from build123d import *

# Parameters (mm, degrees)
PAD001_DEPTH = 2.1
THICKNESS_T  = -0.5
FILLET_R     = 0.3
FILLET001_R  = 0.1


with BuildPart() as part:
    # Sketch001 → Pad001 (new body)
    with BuildSketch(Plane.XY):
        Polygon((5, 18.8), (34, 18.8), (34, 1.2), (1.2, 1.2), (1.2, 15.3), (5, 15.3), align=None)
    extrude(amount=PAD001_DEPTH)

    # Thickness
    thickness_openings = [part.faces().sort_by_distance(p)[0] for p in [
        (17.941945, 9.833744, 0),
    ]]
    offset(amount=THICKNESS_T, openings=thickness_openings, kind=Kind.INTERSECTION)

    # Fillet
    fillet_edges = [part.edges().sort_by_distance(p)[0] for p in [
        (1.2, 1.2, 1.05),
        (34, 1.2, 1.05),
        (34, 18.8, 1.05),
        (5, 18.8, 1.05),
        (5, 15.3, 1.05),
        (1.2, 15.3, 1.05),
        (1.2, 8.25, 2.1),
        (17.6, 1.2, 2.1),
        (34, 10, 2.1),
        (19.5, 18.8, 2.1),
        (5, 17.05, 2.1),
        (3.1, 15.3, 2.1),
    ]]
    fillet(fillet_edges, radius=FILLET_R)

    # Fillet001
    fillet001_edges = [part.edges().sort_by_distance(p)[0] for p in [
        (1.7, 1.7, 0.8),
        (33.5, 1.7, 0.8),
        (33.5, 18.3, 0.8),
        (5.5, 18.3, 0.8),
        (5.5, 14.8, 0.8),
        (1.7, 14.8, 0.8),
        (1.7, 8.25, 1.6),
        (3.6, 14.8, 1.6),
        (5.5, 16.55, 1.6),
        (19.5, 18.3, 1.6),
        (17.6, 1.7, 1.6),
        (33.5, 10, 1.6),
    ]]
    fillet(fillet001_edges, radius=FILLET001_R)


solid = part.part
The listing builds one solid part. Answer for the finished solid, in the listing's coordinates (mm). A direction names the side the tool comes from. Coordinates: 2 decimals unless noted, no trailing zeros. Loops run counter-clockwise (first coordinate to the right, second up) from the corner with the lowest first, then second, coordinate; pieces in that order, holes last. Notation, with made-up numbers: (-15.75, -19) -> (25.25, -19) arc R28 ccw to (25.25, 5) -> close; hole circle Ø7 at (62, 11.5). An arc over 180 degrees is marked (long way). Answer in a Markdown table with one row per item. Add a question column.
1. Consider line 1 (Y direction, x = 20, z = 0.4); line 2 (Y direction, x = 4, z = 0.2); line 3 (X direction, y = 3.5, z = 1.25). Determine where each line is inside the solid, lowest interval first. Write a range as [from, to].
2. For faces 5 (the flat face through (19, 18.3, 1)), 6 (the flat face through (1.2, 8, 1)), determine the directions among +Z, -Z, +X, -X, +Y, -Y from which every point of the face is accessible in a straight line to the end or side of a thin tool.
3. The part is cut by section C-C, the plane y = 6. Write down the section's boundary in (x, z).
4. The part is cut by section B-B, the plane x = 9.5. Write down the section's boundary in (y, z).
5. The part is cut by section A-A, the plane z = 0.7. Write down the section's boundary in (x, y).
6. Determine the mould class of faces 1 (the flat face through (3, 15.3, 1)), 2 (the flat face through (5, 17, 1)), 3 (the flat face through (34, 10, 1)), 4 (the flat face through (33.5, 10, 1)) for opening direction X: +X half, -X half, draft (parallel to the pull), parting line (faces both ways), or undercut.
7. A flat-ended cylindrical pin translates along its axis: P1, Ø1, axis at x = 18, y = 14, coming from the -Z side. Find the tip coordinate at first contact, or state that the pin passes through.
Answer below:
| question | item | result |
|---|---|---|
| 1 | line 1 | [1.2, 1.7], [18.3, 18.8] |
| 1 | line 2 | [1.2, 1.7], [14.8, 15.3] |
| 1 | line 3 | [1.2, 1.7], [33.5, 34] |
| 2 | face 5 | -Z |
| 2 | face 6 | +Z, -Z, -X, +Y, -Y |
| 3 | outline | (1.2, 0) -> (1.7, 0) -> (1.7, 1.5) arc R0.1 cw to (1.8, 1.6) -> (33.4, 1.6) arc R0.1 cw to (33.5, 1.5) -> (33.5, 0) -> (34, 0) -> (34, 1.8) arc R0.3 ccw to (33.7, 2.1) -> (1.5, 2.1) arc R0.3 ccw to (1.2, 1.8) -> close |
| 4 | outline | (1.2, 0) -> (1.7, 0) -> (1.7, 1.5) arc R0.1 cw to (1.8, 1.6) -> (18.2, 1.6) arc R0.1 cw to (18.3, 1.5) -> (18.3, 0) -> (18.8, 0) -> (18.8, 1.8) arc R0.3 ccw to (18.5, 2.1) -> (1.5, 2.1) arc R0.3 ccw to (1.2, 1.8) -> close |
| 5 | outline | (1.2, 1.5) arc R0.3 ccw to (1.5, 1.2) -> (33.7, 1.2) arc R0.3 ccw to (34, 1.5) -> (34, 18.5) arc R0.3 ccw to (33.7, 18.8) -> (5.3, 18.8) arc R0.3 ccw to (5, 18.5) -> (5, 15.6) arc R0.3 cw to (4.7, 15.3) -> (1.5, 15.3) arc R0.3 ccw to (1.2, 15) -> close; hole (1.7, 1.8) arc R0.1 ccw to (1.8, 1.7) -> (33.4, 1.7) arc R0.1 ccw to (33.5, 1.8) -> (33.5, 18.2) arc R0.1 ccw to (33.4, 18.3) -> (5.6, 18.3) arc R0.1 ccw to (5.5, 18.2) -> (5.5, 14.9) arc R0.1 cw to (5.4, 14.8) -> (1.8, 14.8) arc R0.1 ccw to (1.7, 14.7) -> close |
| 6 | face 1 | draft |
| 6 | face 2 | -X half |
| 6 | face 3 | +X half |
| 6 | face 4 | undercut |
| 7 | P1 | z = 1.6 |
